Build history of the part. All positions in model axes, mm. Coordinates: 2 decimals unless noted, no trailing zeros. Order: outer loops, then holes, each group sorted by start corner. A loop starts at its lowest first (then second) coordinate and runs counter-clockwise, first axis right, second up. Notation, with made-up numbers: (11, -36) -> (48, -36) arc R26 cw to (48, 3) -> close; hole circle Ø3 at (-6.5, 65.25). An arc over 180 degrees is marked (long way). Write each question's results on one line, items separated by ' | '.
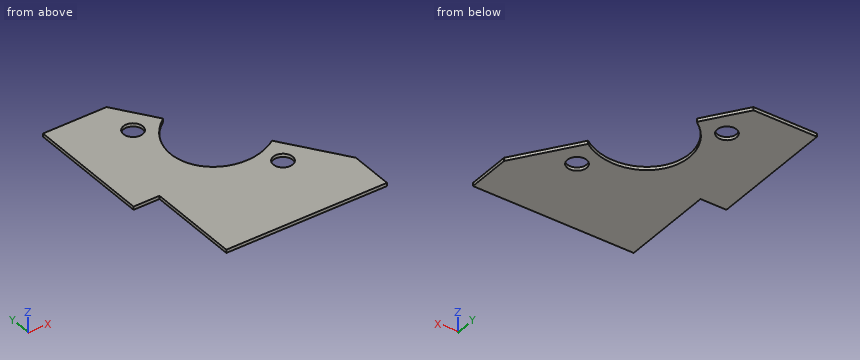
from build123d import *

# Parameters (mm, degrees)
BOSS_EXTRUDE1_DEPTH = 1.5875
SKETCH2_R           = 4.75
CUT_EXTRUDE1_DEPTH  = 135.08080599
CUT_EXTRUDE2_DEPTH  = 135.08080599
SKETCH4_W           = 1.5875
SKETCH4_H           = 62
BOSS_EXTRUDE2_DEPTH = 12.75
SKETCH5_W           = 79
SKETCH5_H           = 1.5875
BOSS_EXTRUDE3_DEPTH = 12.75


with BuildPart() as part:
    # Sketch1 → Boss-Extrude1 (new body)
    with BuildSketch(Plane.XY):
        with BuildLine():
            add(Edge.make_bspline(
                [(32.238440812, 75.351315587), (10.94048766, 60.438328242), (24.132745696, 41.597831224), (37.325003732, 22.757334205), (58.622956884, 37.67032155)],
                knots=[1.570796327, 1.570796327, 1.570796327, 3.141592654, 3.141592654, 4.71238898, 4.71238898, 4.71238898], degree=2, weights=[1, 0.707106781, 1, 0.707106781, 1]))
            Line((58.622956884, 37.67032155), (85, 0))
            Line((85, 0), (0, 0))
            Line((0, 0), (0, 95))
            Line((0, 95), (12.400456604, 103.682893191))
            Line((12.400456604, 103.682893191), (32.238440812, 75.351315587))
        make_face()
    extrude(amount=BOSS_EXTRUDE1_DEPTH)

    # Sketch2 → Cut-Extrude1 (cut, through all)
    with BuildSketch(Plane.XY.offset(1.5875)):
        with Locations((17.813737895, 75.902288156)):
            Circle(SKETCH2_R)
        with Locations((54.207162782, 23.927090946)):
            Circle(SKETCH2_R)
    extrude(amount=-CUT_EXTRUDE1_DEPTH, mode=Mode.SUBTRACT)

    # Sketch3 → Cut-Extrude2 (cut, through all)
    with BuildSketch(Plane.XY.offset(1.5875)):
        Polygon((79, 8.56888804), (79, 0), (85, 0), align=None)
        Polygon((0, 95), (18.48028387, 95), (12.400456604, 103.682893191), align=None)
    extrude(amount=-CUT_EXTRUDE2_DEPTH, mode=Mode.SUBTRACT)

    # Sketch4 → Boss-Extrude2 (add)
    with BuildSketch(Plane.ZY):
        with Locations((0.79375, 64)):
            Rectangle(SKETCH4_W, SKETCH4_H)
    extrude(amount=BOSS_EXTRUDE2_DEPTH)

    # Sketch5 → Boss-Extrude3 (add)
    with BuildSketch(Plane.XZ):
        with Locations((39.5, 0.79375)):
            Rectangle(SKETCH5_W, SKETCH5_H)
    extrude(amount=BOSS_EXTRUDE3_DEPTH)


solid = part.part
Item 1: Slice it at D-D, the plane x = 67.5. List the corners of the cut face in (y, z), and give its area (3 significant figures).
Answer:
outline: (-12.75, 0) -> (24.99, 0) -> (24.99, 1.59) -> (-12.75, 1.59) -> close | area: 59.9 mm^2
Item 2: Slice it at A-A, the plane y = 22.5. List the corners of the cut face in (x, z).
Answer:
outline: (0, 0) -> (49.68, 0) -> (49.68, 1.59) -> (0, 1.59) -> close; (58.74, 0) -> (69.25, 0) -> (69.25, 1.59) -> (58.74, 1.59) -> close
Item 3: Slice it at C-C, the plane z = 1.3. State how many separate pieces and enclosed holes the cut face has, and give its area (3 significant figures).
Answer:
separate pieces: 1 | enclosed holes: 2 | area: 5,610 mm^2
Item 4: Pin check, flat tips, straight feed: pin 1 (15 mm diameter, centred on x = 54.21, y = 23.93, fed in from -Z); pin 2 (0.8 mm diameter, centred on y = 8, z = 0.5, fed in from -X); pin 3 (6 mm diameter, centred on x = 57, y = 43, fed in from +Z). Stop position of each tip, or through.
Answer:
pin 1: stops at z = 0 | pin 2: stops at x = 0 | pin 3: passes through
Item 5: Drill centre lines: line 1 (Y direction, x = 55, z = 1.5); line 2 (X direction, y = 20, z = 0.8) (3 decimals); line 3 (X direction, y = 21, z = 1.35). Where is each one in solid material? Low to high. Write a range as from..to.
Answer:
line 1: y = -12.75..19.24, 28.61..35.5 | line 2: x = 0..51.535, 56.879..70.996 | line 3: x = 0..50.47, 57.95..70.3
Item 6: Slice it at B-B, the plane x = 15.5. List the corners of the cut face in (y, z).
Answer:
outline: (-12.75, 0) -> (71.75, 0) -> (71.75, 1.59) -> (-12.75, 1.59) -> close; (80.05, 0) -> (95, 0) -> (95, 1.59) -> (80.05, 1.59) -> close
